from build123d import *

# Parameters (mm, degrees)
BOSS_EXTRUDE1_DEPTH      = 225
BOSS_EXTRUDE1_DEPTH_BACK = 225
FILLET1_R                = 13.5
FILLET2_R                = 13.5
FILLET3_R                = 13.5


with BuildPart() as part:
    # Sketch1 → Boss-Extrude1 (new, two sides: drawn at the far end of the back side and taken through both)
    with BuildSketch(Plane.XY.offset(-BOSS_EXTRUDE1_DEPTH_BACK)):
        with BuildLine():
            Line((-329.1, -55), (-329.1, -80))
            Line((-329.1, -80), (-156.365701077, -80))
            ThreePointArc((-156.365701077, -80), (-147.072914305, -76.292554009), (-142.884202358, -67.206535409))
            Line((-142.884202358, -67.206535409), (-139.982869184, -11.845800547))
            ThreePointArc((-139.982869184, -11.845800547), (-136.104432196, -3.432820362), (-127.5, 0))
            Line((-127.5, 0), (127.5, 0))
            ThreePointArc((127.5, 0), (136.104432196, -3.432820362), (139.982869184, -11.845800547))
            Line((139.982869184, -11.845800547), (142.884202358, -67.206535409))
            ThreePointArc((142.884202358, -67.206535409), (147.072914305, -76.292554009), (156.365701077, -80))
            Line((156.365701077, -80), (329.1, -80))
            Line((329.1, -80), (329.1, -55))
            Line((329.1, -55), (179.140850678, -55))
            ThreePointArc((179.140850678, -55), (170.536418482, -51.567179638), (166.657981494, -43.154199453))
            Line((166.657981494, -43.154199453), (163.75664832, 12.206535409))
            ThreePointArc((163.75664832, 12.206535409), (159.567936373, 21.292554009), (150.275149601, 25))
            Line((150.275149601, 25), (-150.275149601, 25))
            ThreePointArc((-150.275149601, 25), (-159.567936373, 21.292554009), (-163.75664832, 12.206535409))
            Line((-163.75664832, 12.206535409), (-166.657981494, -43.154199453))
            ThreePointArc((-166.657981494, -43.154199453), (-170.536418482, -51.567179638), (-179.140850678, -55))
            Line((-179.140850678, -55), (-329.1, -55))
        make_face()
    extrude(amount=BOSS_EXTRUDE1_DEPTH + BOSS_EXTRUDE1_DEPTH_BACK)

    # Fillet1
    fillet1_edges = [part.edges().sort_by_distance(p)[0] for p in [
        (-242.732850539, -80, -225),
        (-147.072914305, -76.292554009, -225),
        (-141.433535771, -39.526167978, -225),
        (-136.104432196, -3.432820362, -225),
        (0, 0, -225),
        (136.104432196, -3.432820362, -225),
        (-329.1, -80, 0),
        (141.433535771, -39.526167978, -225),
        (147.072914305, -76.292554009, -225),
        (242.732850539, -80, -225),
        (-242.732850539, -80, 225),
        (-147.072914305, -76.292554009, 225),
        (-141.433535771, -39.526167978, 225),
        (-136.104432196, -3.432820362, 225),
        (0, 0, 225),
        (136.104432196, -3.432820362, 225),
        (141.433535771, -39.526167978, 225),
        (147.072914305, -76.292554009, 225),
        (242.732850539, -80, 225),
    ]]
    fillet(fillet1_edges, radius=FILLET1_R)

    # Fillet2
    fillet2_edges = [part.edges().sort_by_distance(p)[0] for p in [
        (329.1, -80, 0),
        (329.1, -60.75, 225),
        (329.1, -60.75, -225),
        (329.1, -76.045941546, 221.045941546),
        (329.1, -76.045941546, -221.045941546),
    ]]
    fillet(fillet2_edges, radius=FILLET2_R)

    # Fillet3
    # the kernel refuses this fillet: 13.5 mm, written as the material it takes off along each edge
    with BuildSketch(Plane(origin=(-315.6, -66.5, 211.5), x_dir=(0, 0, 1), z_dir=(-1, 0, 0))) as fillet3_piece_1_section:
        Polygon((0, 0), (FILLET3_R, 0), (FILLET3_R, -FILLET3_R), (0, -FILLET3_R), align=None)
    fillet3_piece_1 = extrude(amount=FILLET3_R, mode=Mode.PRIVATE)
    fillet3_piece_1 = fillet3_piece_1 - Plane(origin=(-315.6, -66.5, 211.5), x_dir=(0, 0.7071067811865475, -0.7071067811865475), z_dir=(-1, 0, 0)) * Sphere(FILLET3_R, mode=Mode.PRIVATE)
    add(fillet3_piece_1, mode=Mode.SUBTRACT)
    with BuildSketch(Plane(origin=(-315.6, -66.5, -211.5), x_dir=(-1, 0, 0), z_dir=(0, 0, -1))) as fillet3_piece_2_section:
        Polygon((0, 0), (FILLET3_R, 0), (FILLET3_R, -FILLET3_R), (0, -FILLET3_R), align=None)
    fillet3_piece_2 = extrude(amount=FILLET3_R, mode=Mode.PRIVATE)
    fillet3_piece_2 = fillet3_piece_2 - Plane(origin=(-315.6, -66.5, -211.5), x_dir=(0.7071067811865475, 0.7071067811865475, 0), z_dir=(0, 0, -1)) * Sphere(FILLET3_R, mode=Mode.PRIVATE)
    add(fillet3_piece_2, mode=Mode.SUBTRACT)
    with BuildSketch(Plane(origin=(-329.1, -21.25, 225), x_dir=(0, 0, -1), z_dir=(0, -1, 0)), Plane(origin=(-329.1, -21.25, -225), x_dir=(1, 0, 0), z_dir=(0, -1, 0))) as fillet3_piece_3:
        with BuildLine():
            CenterArc((FILLET3_R, FILLET3_R), FILLET3_R, 180, 90)
            Line((0, FILLET3_R), (0, 0))
            Line((0, 0), (FILLET3_R, 0))
        make_face()
    extrude(amount=45.25, mode=Mode.SUBTRACT)


solid = part.part
Model file for the job. Use its own axes, mm. A direction names the side the tool comes from. Give positions to 0.01 mm unless a question says otherwise; leave off trailing zeros. Order: outer loops, then holes, each group sorted by start corner. A loop starts at its lowest first (then second) coordinate and runs counter-clockwise, first axis right, second up. Notation, with made-up numbers: (-35, 81) - (-9, 81) arc R23 cw to (-9, 117) - close; hole circle Ø10 at (23.5, 67.25). An arc over 180 degrees is marked (long way). Write item = value, one per line. Start each with the question number.
1. Probe line 1 along X through (y, z) = (-66.5, -158.5); line 2 along Y through (x, z) = (-273.5, -157); line 3 along Y through (x, z) = (64, -107.5). List the from-to ranges inside material, lowest first.
2. Cut at A-A, the plane z = -171. List the corners of the cut face in (x, y), and give its area (3 significant figures).
3. Two-plate mould, pull along X, no slides. Class faces 6 (the cylindrical face through (1.78, 3.85, -220.94)), 7 (the flat face through (-2, 0, -3)), 8 (the cylindrical face through (237.1, -76.15, -220.94)), 9 (the cylindrical face through (325.25, -60.83, -220.94)): pulls with the +X half, pulls with the -X half, needs draft (parallel to the pull), parting line crosses it, or undercut.
4. Drop flat-ended pins along their axis: P1, Ø4, axis at x = -71, y = 5, coming from the -Z side; P2, Ø8, axis at y = -27.5, z = 142, coming from the +X side; P3, Ø3, axis at y = -48, z = -8, coming from the -X side. Give the stop position or say it passes through.
5. Which spindle directions (+Z, -Z, +X, -X, +Y, -Y) get a long thin tool onto all of the face, cutting with end or side? Do faces 1 (the flat face through (-253, -55, -3)), 2 (the flat face through (-141.454, -39.914, -2.961)), 3 (the cylindrical face through (-145.26, -38.94, -220.94)), 4 (the cylindrical face through (1.78, 3.85, 220.94)), 5 (the flat face through (255, -55, -3)). Say none if no direction does.
6. Cut at B-B, the plane x = 83.5. List the corners of the cut face in (y, z).
Taken from the geometry:
q1.line_1 = -329.1 to -142.85, 142.85 to 329.1
q1.line_2 = -80 to -55
q1.line_3 = 0 to 25
q2.outline = (-329.1, -66.5) arc R13.5 ccw to (-315.6, -80) - (-156.37, -80) arc R13.5 ccw to (-142.88, -67.21) - (-139.98, -11.85) arc R12.5 cw to (-127.5, 0) - (127.5, 0) arc R12.5 cw to (139.98, -11.85) - (142.88, -67.21) arc R13.5 ccw to (156.37, -80) - (315.6, -80) arc R13.5 ccw to (329.1, -66.5) - (329.1, -55) - (179.14, -55) arc R12.5 cw to (166.66, -43.15) - (163.76, 12.21) arc R13.5 ccw to (150.28, 25) - (-150.28, 25) arc R13.5 ccw to (-163.76, 12.21) - (-166.66, -43.15) arc R12.5 cw to (-179.14, -55) - (-329.1, -55) - close
q2.area = 20,200 mm²
q3.face_6 = undercut
q3.face_7 = undercut
q3.face_8 = needs draft
q3.face_9 = pulls with the +X half
q4.P1 = -223.33
q4.P2 = 166.05
q4.P3 = -168.78
q5.face_1 = +Z, -Z, -X, +Y
q5.face_2 = +Z, -Z, -Y
q5.face_3 = -Z, -Y
q5.face_4 = +Z, -Y
q5.face_5 = +Z, -Z, +X, +Y
q6.outline = (0, -211.5) arc R13.5 ccw to (13.5, -225) - (25, -225) - (25, 225) - (13.5, 225) arc R13.5 ccw to (0, 211.5) - close
